Build history of the part. All positions in model axes, mm. Give positions to 0.01 mm unless a question says otherwise; leave off trailing zeros. Loops run counter-clockwise (first coordinate to the right, second up) from the corner with the lowest first, then second, coordinate; pieces in that order, holes last. Notation, with made-up numbers: (86.5, -2) -> (127.5, -2) arc R19 cw to (127.5, 21) -> close; hole circle Ø1 at (-26, 4.5). An arc over 180 degrees is marked (long way). Answer as a JSON object with one key per item and string values. Group by question number.
Q1. Band-saw the part on A-A, the plane x = -3. Write the cut outline in (y, z) (3 decimals), plus the area to 3 significant figures.
Q2. Drop a flat-ended pin along its axis: pin 1 (1 mm diameter, centred on y = -32.5, z = -1, fed in from +X). Give the stop position or say it passes through.
Q3. Band-saw the part on B-B, the plane z = -1.75. Write the cut outline in (x, y) (3 decimals), plus the area to 3 significant figures.
Q4. Wall check: probe 1 along Y at (x, z) = (5, -0.65) (3 decimals); probe 2 along X at (y, z) = (-32.5, -1) (3 decimals); probe 3 along Y at (x, z) = (33, -1.55). Give the ranges that are in metal, low to high. Write a range as from..to.
from build123d import *

# Parameters (mm, degrees)
F0_W     = 19.05
F0_H     = 3.175
F1_DEPTH = 3.175


# Not quite as in the source:
# - a length typed as a fraction of an inch, garbled in the dataset ("3 / 203.2 mm" for 3/8 in), is restored


with BuildPart() as f1:
    # F0 (on Top) → F1 (new body)
    with BuildSketch(Plane.XY):
        with BuildLine():
            Line((31.75, 38.1), (-31.75, 38.1))
            ThreePointArc((-31.75, 38.1), (-36.2401280605, 36.2401280605), (-38.1, 31.75))
            Line((-38.1, 31.75), (-38.1, -31.75))
            ThreePointArc((-38.1, -31.75), (-36.2401280605, -36.2401280605), (-31.75, -38.1))
            Line((-31.75, -38.1), (31.75, -38.1))
            ThreePointArc((31.75, -38.1), (36.2401280605, -36.2401280605), (38.1, -31.75))
            Line((38.1, -31.75), (38.1, 31.75))
            ThreePointArc((38.1, 31.75), (36.2401280605, 36.2401280605), (31.75, 38.1))
        make_face()
        with Locations((0, -33.3375)):
            Rectangle(F0_W, F0_H, mode=Mode.SUBTRACT)
        with Locations((0, 33.3375)):
            Rectangle(F0_W, F0_H, mode=Mode.SUBTRACT)
    extrude(amount=-F1_DEPTH)


solid = f1.part
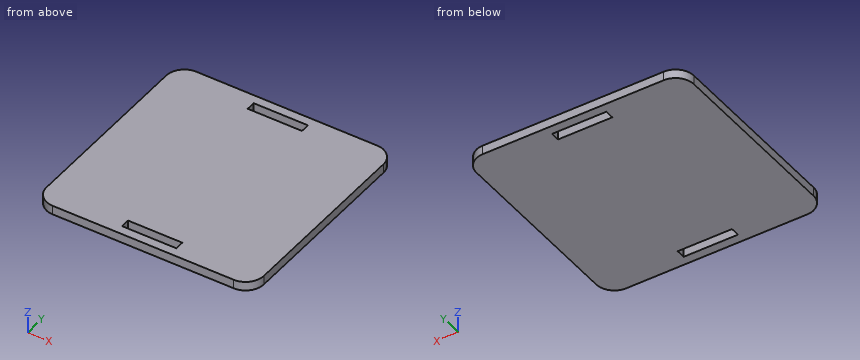
Worked answers:
{
 "1": {"outline": "(-38.1, -3.175) -> (-34.925, -3.175) -> (-34.925, 0) -> (-38.1, 0) -> close; (-31.75, -3.175) -> (31.75, -3.175) -> (31.75, 0) -> (-31.75, 0) -> close; (34.925, -3.175) -> (38.1, -3.175) -> (38.1, 0) -> (34.925, 0) -> close", "area": "222 mm2"},
 "2": {"pin 1": "x = 38.1"},
 "3": {"outline": "(-38.1, -31.75) arc R6.35 ccw to (-31.75, -38.1) -> (31.75, -38.1) arc R6.35 ccw to (38.1, -31.75) -> (38.1, 31.75) arc R6.35 ccw to (31.75, 38.1) -> (-31.75, 38.1) arc R6.35 ccw to (-38.1, 31.75) -> close; hole (-9.525, -34.925) -> (9.525, -34.925) -> (9.525, -31.75) -> (-9.525, -31.75) -> close; hole (-9.525, 31.75) -> (9.525, 31.75) -> (9.525, 34.925) -> (-9.525, 34.925) -> close", "area": "5,650 mm2"},
 "4": {"probe 1": "-38.1..-34.925, -31.75..31.75, 34.925..38.1", "probe 2": "-38.056..-9.525, 9.525..38.056", "probe 3": "-37.98..37.98"}
}
